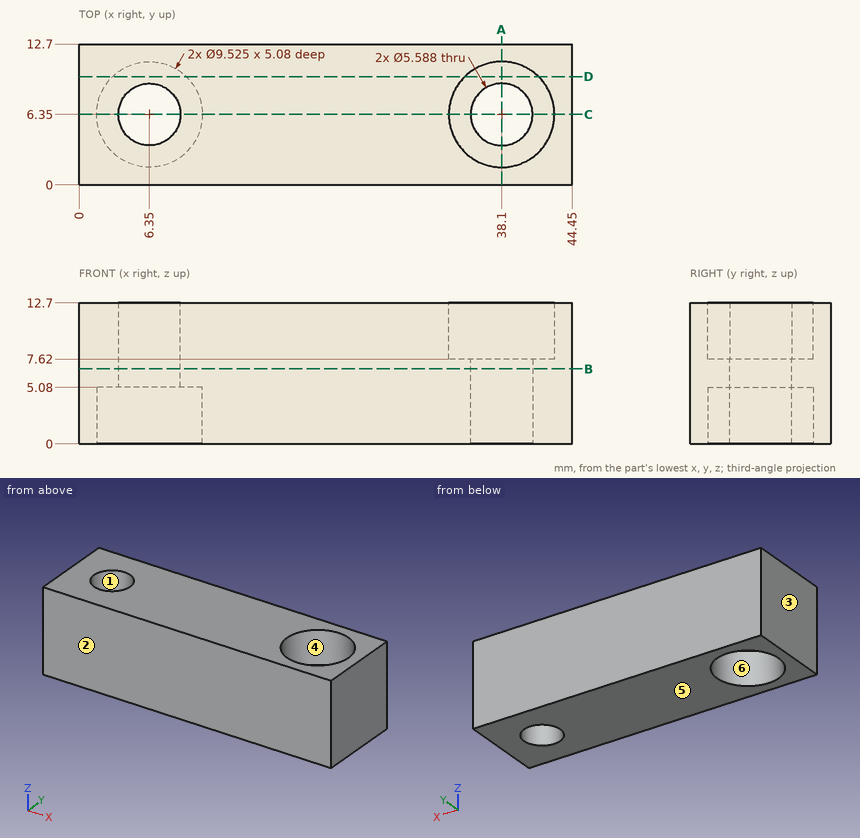
Study the drawing (mm; zero at the part's minimum x, y, z) and answer. A direction names the side the tool comes from. Give positions to 0.01 mm unless a question says otherwise; leave off trailing zeros. Write each loop counter-clockwise with the first axis right and the second up, starting at its lowest first coordinate (ties: lowest second). Pieces come first, ordered by that corner, then holes.
(1) The part is cut by section D-D on y = 9.75. Write down the section's boundary in (x, z).
Final values:
outline: (0, 0) - (3.02, 0) - (3.02, 5.08) - (9.68, 5.08) - (9.68, 0) - (44.45, 0) - (44.45, 12.7) - (41.43, 12.7) - (41.43, 7.62) - (34.77, 7.62) - (34.77, 12.7) - (0, 12.7) - close
(2) The mould has two halves that part along Y. Classify the marked faces 1, 2 and 3: pulls with the +Y half, pulls with the -Y half, needs draft (parallel to the pull), parting line crosses it, or undercut.
Final values:
face 1: undercut
face 2: pulls with the -Y half
face 3: needs draft
(3) The part is cut by section A-A on x = 38.1. Write down the section's boundary in (y, z).
Final values:
outline: (0, 0) - (3.56, 0) - (3.56, 7.62) - (1.59, 7.62) - (1.59, 12.7) - (0, 12.7) - close; (9.14, 0) - (12.7, 0) - (12.7, 12.7) - (11.11, 12.7) - (11.11, 7.62) - (9.14, 7.62) - close
(4) The part is cut by section B-B on z = 6.75. Write down the section's boundary in (x, y).
Final values:
outline: (0, 0) - (44.45, 0) - (44.45, 12.7) - (0, 12.7) - close; hole circle Ø5.59 at (6.35, 6.35); hole circle Ø5.59 at (38.1, 6.35)
(5) Flat-ended cylindrical pins translate along their axes: pin 1 Ø2 at (y, z) = (7, 8.5) entering from -X; pin 2 Ø5 at (x, y) = (37.5, 6.5) entering from +Z; pin 3 Ø1.5 at (x, y) = (8.5, 4) entering from -Z; pin 4 Ø3.5 at (x, y) = (38.1, 6.35) entering from +Z. Find the tip coordinate at first contact, or state that the pin passes through.
Final values:
pin 1: stops at x = 0
pin 2: stops at z = 7.62
pin 3: stops at z = 5.08
pin 4: passes through
(6) Straight lines are drawn through the part: line 1 (X direction, y = 6.5, z = 2.75); line 2 (Y direction, x = 6.35, z = 3.55); line 3 (Y direction, x = 38.1, z = 2.5). For each, find the intervals that lie inside material, in ascending order.
Final values:
line 1: x = 0 to 1.59, 11.11 to 35.31, 40.89 to 44.45
line 2: y = 0 to 1.59, 11.11 to 12.7
line 3: y = 0 to 3.56, 9.14 to 12.7
(7) The part is cut by section C-C on y = 6.35. Write down the section's boundary in (x, z), plus the area to 3 significant figures.
Final values:
outline: (0, 0) - (1.59, 0) - (1.59, 5.08) - (3.56, 5.08) - (3.56, 12.7) - (0, 12.7) - close; (9.14, 5.08) - (11.11, 5.08) - (11.11, 0) - (35.31, 0) - (35.31, 7.62) - (33.34, 7.62) - (33.34, 12.7) - (9.14, 12.7) - close; (40.89, 0) - (44.45, 0) - (44.45, 12.7) - (42.86, 12.7) - (42.86, 7.62) - (40.89, 7.62) - close
area: 383 mm2
(8) Which of the six approach directions +Z, -Z, +X, -X, +Y, -Y give full straight-line access (tool end or side, diameter ignored) to the marked faces 4, 5 and 6?
Final values:
face 4: +Z
face 5: -Z, +X, -X, +Y, -Y
face 6: -Z
